```python
from build123d import *

# Parameters (mm, degrees)
SKETCH1_R                  = 3.75
BOSS_EXTRUDE1_DEPTH        = 10.5
F_3_5_3_5_DIAMETER_HOLE1_D = 3.5
SKETCH4_R                  = 4.75
BOSS_EXTRUDE2_DEPTH        = 3.5


with BuildPart() as part:
    # Sketch1 → Boss-Extrude1 (new body)
    with BuildSketch(Plane(origin=(0, 0, 0), x_dir=(1, 0, 0), z_dir=(0, 1, 0))):
        with Locations(Location((0, 0, 0), (0, 0, 90))):
            Circle(SKETCH1_R)
    extrude(amount=BOSS_EXTRUDE1_DEPTH)

    # Ø3.5 (3.5) Diameter Hole1 (through all)
    with Locations(Plane(origin=(0, 10.5, 0), x_dir=(1, 0, 0), z_dir=(0, 1, 0))):
        with Locations((0, 0)):
            Hole(F_3_5_3_5_DIAMETER_HOLE1_D / 2)

    # Sketch4 → Boss-Extrude2 (add)
    with BuildSketch(Plane.XZ):
        with Locations(Location((0, 0, 0), (0, 0, 270))):
            Circle(SKETCH4_R)
    extrude(amount=-BOSS_EXTRUDE2_DEPTH)


solid = part.part
```
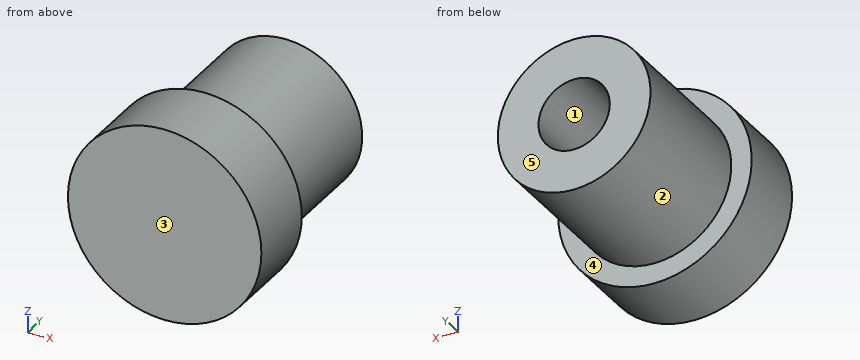
Could you check a few things on this model? Use its own coordinates, in mm. Face numbers are marked on the shaded views. A direction names the side the tool comes from. Coordinates: 2 decimals unless noted, no trailing zeros. Write each loop counter-clockwise with the first axis right and the second up, starting at its lowest first coordinate (ties: lowest second). Pieces come first, ordered by that corner, then holes. Notation, with made-up numbers: (25.25, 35) -> (71.25, 35) arc R34 ccw to (71.25, 65) -> close; hole circle Ø2 at (-35, 57.25). An arc over 180 degrees is marked (long way). One line per question, with ' | ' between items. Start each with the question number.
1. If we section it at A-A (x = 0): Please give me the cut outline in (y, z), and give its area (4 significant figures).
2. Will these pins go through, and if not, where does the flat tip stop? P1, Ø2, axis at x = 0, z = 0, coming from the +Y side; P2, Ø4, axis at y = 6, z = -3, coming from the -X side.
3. If we section it at C-C (y = 9): Please give me the cut outline in (x, z), and give its area (3 significant figures).
4. Thinking about a two-plate mould opening in X: for the marked faces 1, 2 and 3, which applies, pulls with the +X half, pulls with the -X half, needs draft (parallel to the pull), parting line crosses it, or undercut?
5. For the marked faces 4 and 5, which set-ups out of +Z, -Z, +X, -X, +Y, -Y let a thin tool reach every point of the face, with its end or its side?
6. Please list where these lines run through material, in increasing order: line 1 along Y through (x, z) = (1.5, -4); line 2 along X through (y, z) = (3.75, 1); line 3 along X through (y, z) = (7.75, -1.25).
7. If we section it at B-B (z = 0): Please give me the cut outline in (x, y), and give its area (4 significant figures).
8. If we section it at D-D (z = 2.75): Please give me the cut outline in (x, y).
Return value:
1) outline: (0, -4.75) -> (3.5, -4.75) -> (3.5, -3.75) -> (10.5, -3.75) -> (10.5, -1.75) -> (3.5, -1.75) -> (3.5, 1.75) -> (10.5, 1.75) -> (10.5, 3.75) -> (3.5, 3.75) -> (3.5, 4.75) -> (0, 4.75) -> close | area: 61.25 mm²
2) P1: stops at y = 3.5 | P2: stops at x = -3.61
3) outline: circle Ø7.5 at (0, 0); hole circle Ø3.5 at (0, 0) | area: 34.6 mm²
4) face 1: undercut | face 2: parting line crosses it | face 3: needs draft
5) face 4: +Y | face 5: +Z, -Z, +X, -X, +Y
6) line 1: y = 0 to 3.5 | line 2: x = -3.61 to -1.44, 1.44 to 3.61 | line 3: x = -3.54 to -1.22, 1.22 to 3.54
7) outline: (-4.75, 0) -> (4.75, 0) -> (4.75, 3.5) -> (3.75, 3.5) -> (3.75, 10.5) -> (1.75, 10.5) -> (1.75, 3.5) -> (-1.75, 3.5) -> (-1.75, 10.5) -> (-3.75, 10.5) -> (-3.75, 3.5) -> (-4.75, 3.5) -> close | area: 61.25 mm²
8) outline: (-3.87, 0) -> (3.87, 0) -> (3.87, 3.5) -> (2.55, 3.5) -> (2.55, 10.5) -> (-2.55, 10.5) -> (-2.55, 3.5) -> (-3.87, 3.5) -> close
